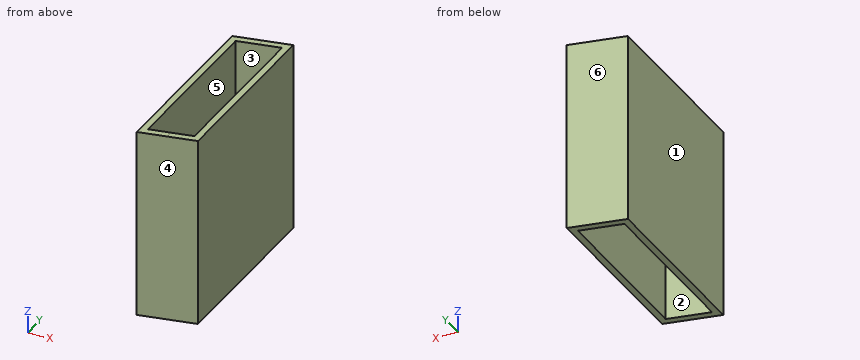
```python
from build123d import *

# Parameters (mm, degrees)
SKETCH2_W               = 9.652
SKETCH2_H               = 3.048
SKETCH2_W_2             = 3.048
SKETCH2_H_2             = 35.052
BOSS_EXTRUDE1_DEPTH     = 78.985121
SKETCH5_W               = 25.4
SKETCH5_H               = 76.2
SKETCH5_W_2             = 19.304
SKETCH5_H_2             = 70.104
BOSS_EXTRUDE3_DEPTH     = 50
CUT_EXTRUDE1_DEPTH      = 1
CUT_EXTRUDE1_DEPTH_BACK = 77.2
SKETCH7_W               = 25.4
SKETCH7_H               = 76.2
SKETCH7_W_2             = 19.304
SKETCH7_H_2             = 70.104
BOSS_EXTRUDE4_DEPTH     = 50
CUT_EXTRUDE2_DEPTH      = 1
CUT_EXTRUDE2_DEPTH_BACK = 77.2


with BuildPart() as part:
    # Sketch2 → Boss-Extrude1 (new body)
    with BuildSketch(Plane.XY):
        Polygon((-12.7, 0), (-9.652, 0), (-9.652, 35.052), (-9.652, 38.1), (-12.7, 38.1), align=None)
        with Locations((-4.826, 36.576)):
            Rectangle(SKETCH2_W, SKETCH2_H)
        Polygon((0, 38.1), (0, 35.052), (9.652, 35.052), (9.652, 0), (12.7, 0), (12.7, 38.1), align=None)
        with Locations((11.176, -17.526)):
            Rectangle(SKETCH2_W_2, SKETCH2_H_2)
        Polygon((-9.652, -35.052), (-9.652, 0), (-12.7, 0), (-12.7, -38.1), (0, -38.1), (0, -35.052), align=None)
        Polygon((9.652, -35.052), (0, -35.052), (0, -38.1), (12.7, -38.1), (12.7, -35.052), align=None)
    extrude(amount=BOSS_EXTRUDE1_DEPTH)

    # Sketch5 → Boss-Extrude3 (add)
    with BuildSketch(Plane(origin=(0, 0, 0), x_dir=(-1, 0, 0), z_dir=(0, 0, -1))):
        Rectangle(SKETCH5_W, SKETCH5_H)
        Rectangle(SKETCH5_W_2, SKETCH5_H_2, mode=Mode.SUBTRACT)
    extrude(amount=BOSS_EXTRUDE3_DEPTH)

    # Sketch6 → Cut-Extrude1 (cut, two sides)
    with BuildSketch(Plane.XZ.offset(38.1)) as cut_extrude1_sk:
        Polygon((-12.7, -1.617644511), (-45.228253893, -5.760884774), (-37.756637, -64.41996217), (45.640291612, -53.797396519), (38.168674718, 4.861680877), (12.7, -48.058587426), (12.7, -50), (-12.7, -50), align=None)
        Polygon((0, 0), (-12.7, -1.617644511), (-12.7, -50), (12.7, -50), (12.7, -48.058587426), (12.534006261, -48.403498707), align=None)
        Polygon((38.168674718, 4.861680877), (12.7, 1.617644511), (12.7, -48.058587426), align=None)
        Polygon((12.7, 1.617644511), (0, 0), (12.534006261, -48.403498707), (12.7, -48.058587426), align=None)
    extrude(amount=CUT_EXTRUDE1_DEPTH, mode=Mode.SUBTRACT)
    extrude(cut_extrude1_sk.sketch, amount=-CUT_EXTRUDE1_DEPTH_BACK, mode=Mode.SUBTRACT)

    # Sketch7 → Boss-Extrude4 (add)
    with BuildSketch(Plane.XY.offset(78.985120912)):
        Rectangle(SKETCH7_W, SKETCH7_H)
        Rectangle(SKETCH7_W_2, SKETCH7_H_2, mode=Mode.SUBTRACT)
    extrude(amount=BOSS_EXTRUDE4_DEPTH)

    # Sketch8 → Cut-Extrude2 (cut, two sides)
    with BuildSketch(Plane(origin=(0, 38.1, 0), x_dir=(1, 0, 0), z_dir=(0, 1, 0))) as cut_extrude2_sk:
        Polygon((-12.534006261, -127.388619619), (-12.7, -126.667826545), (-12.7, -128.985120912), (12.7, -128.985120912), (12.7, -80.602765422), (0, -78.985120912), align=None)
        Polygon((-12.7, -77.367476401), (-24.396635689, -75.877633998), (-12.7, -126.667826545), align=None)
        Polygon((0, -78.985120912), (-12.7, -77.367476401), (-12.7, -126.667826545), (-12.534006261, -127.388619619), align=None)
    extrude(amount=CUT_EXTRUDE2_DEPTH, mode=Mode.SUBTRACT)
    extrude(cut_extrude2_sk.sketch, amount=-CUT_EXTRUDE2_DEPTH_BACK, mode=Mode.SUBTRACT)


solid = part.part
```
Read the model definition and answer for the solid it produces. Units are mm, in the model's axes. Face numbers are marked on the shaded views. A direction names the side the tool comes from. Coordinates: 2 decimals unless noted, no trailing zeros. Write each loop counter-clockwise with the first axis right and the second up, starting at its lowest first coordinate (ties: lowest second). Pieces come first, ordered by that corner, then holes. Notation, with made-up numbers: (18.5, 48.5) - (50.5, 48.5) arc R21 ccw to (50.5, 83.5) - close; hole circle Ø10 at (48, -26.5). An arc over 180 degrees is marked (long way). Answer as a JSON object with one key per item and string values. Group by question number.
1. A cutting plane is placed at B-B (y = -2.5). Determine the outline of the cut face in (x, z), plus the area to 3 significant figures.
2. A cutting plane is placed at A-A (z = 40.5). Determine the outline of the cut face in (x, y), plus the area to 3 significant figures.
3. The mould has two halves that part along Y. Classify the marked faces 1, 2, 3 and 4: +Y half, -Y half, draft (parallel to the pull), parting line (faces both ways), or undercut.
4. Consider L1, parallel to X at y = 19.5, z = 68; L2, parallel to Y at x = 2, z = 27; L3, parallel to Z at x = 9.75, y = -14. Determine where each line is inside the solid, lowest interval first. Write a range as [from, to].
5. A cutting plane is placed at C-C (x = -2.25). Determine the outline of the cut face in (y, z).
6. Each of these flat-tipped pins is pushed along its axis until it touches: P1, Ø3, axis at x = -8, y = 13.5, coming from the +Z side; P2, Ø12, axis at x = 8, y = -28.5, coming from the +Z side. Where does it stop, or does it pass through?
7. Which of the six approach directions +Z, -Z, +X, -X, +Y, -Y give full straight-line access (tool end or side, diameter ignored) to the marked faces 5 and 6?
Worked out:
{
 "1": {"outline": "(-12.7, -1.62) - (-9.65, -1.23) - (-9.65, 77.76) - (-12.7, 77.37) - close; (9.65, 1.23) - (12.7, 1.62) - (12.7, 80.6) - (9.65, 80.21) - close", "area": "481 mm²"},
 "2": {"outline": "(-12.7, -38.1) - (12.7, -38.1) - (12.7, 38.1) - (-12.7, 38.1) - close; hole (-9.65, -35.05) - (9.65, -35.05) - (9.65, 35.05) - (-9.65, 35.05) - close", "area": "582 mm²"},
 "3": {"face 1": "draft", "face 2": "undercut", "face 3": "undercut", "face 4": "-Y half"},
 "4": {"L1": "x = [-12.7, -9.65], [9.65, 12.7]", "L2": "y = [-38.1, -35.05], [35.05, 38.1]", "L3": "z = [1.24, 80.23]"},
 "5": {"outline": "(-38.1, -0.29) - (-35.05, -0.29) - (-35.05, 78.7) - (-38.1, 78.7) - close; (35.05, -0.29) - (38.1, -0.29) - (38.1, 78.7) - (35.05, 78.7) - close"},
 "6": {"P1": "passes through", "P2": "stops at z = 80.6"},
 "7": {"face 5": "+Z, -Z", "face 6": "+Z, -Z, +X, -X, +Y"}
}
